Can you work these out from the model? Positions are in its coordinate system, mm. A direction names the side the tool comes from. Round coordinates to 2 decimals unless told otherwise and drop trailing zeros. Order: outer loops, then holes, each group sorted by start corner. A loop starts at its lowest first (then second) coordinate and runs counter-clockwise, first axis right, second up.
from build123d import *

# Parameters (mm, degrees)
EXTRUDE_1_DEPTH      = 12
EXTRUDE_1_DEPTH_BACK = 12
SKETCH_1_W           = 130
SKETCH_1_H           = 112
SKETCH_2_W           = 10.341275007
SKETCH_2_H           = 108.506204724
CUT_EXTRUDE_1_DEPTH  = 90.089842294
SKETCH_3_W           = 108.506204724
SKETCH_3_H           = 4.039795579
SKETCH_3_H_2         = 16.032937215
CUT_EXTRUDE_2_DEPTH  = 5
CHAMFER_1_SIZE       = 5
FILLET_1_R           = 5
CHAMFER_2_SIZE       = 2.747477419
CHAMFER_2_SIZE_2     = 1
FILLET_2_R           = 2
SKETCH_4_W           = 9.4
SKETCH_4_H           = 11
SKETCH_4_W_2         = 7.4
SKETCH_4_H_2         = 9
EXTRUDE_2_DEPTH      = 8
SKETCH_5_W           = 122.805441914
SKETCH_5_H           = 111.758877205
CUT_EXTRUDE_3_DEPTH  = 2


with BuildPart() as part:
    # 草图1 → 凸台-拉伸1 (new, two sides: drawn at the far end of the back side and taken through both)
    with BuildSketch(Plane(origin=(0, 0, 0), x_dir=(1, 0, 0), z_dir=(0, 1, 0)).offset(-EXTRUDE_1_DEPTH_BACK)):
        Rectangle(SKETCH_1_W, SKETCH_1_H)
    extrude(amount=EXTRUDE_1_DEPTH + EXTRUDE_1_DEPTH_BACK)

    # 草图2 → 切除-拉伸1 (cut, through all)
    with BuildSketch(Plane(origin=(0, 12, 0), x_dir=(1, 0, 0), z_dir=(0, 1, 0))):
        with Locations((59.829362496, 1.746897638)):
            Rectangle(SKETCH_2_W, SKETCH_2_H)
        with Locations((-59.829362496, 1.746897638)):
            Rectangle(SKETCH_2_W, SKETCH_2_H)
    extrude(amount=-CUT_EXTRUDE_1_DEPTH, mode=Mode.SUBTRACT)

    # 草图3 → 切除-拉伸2 (cut)
    with BuildSketch(Plane.ZY.offset(54.658724993)):
        with Locations((-1.746897638, 9.980102211)):
            Rectangle(SKETCH_3_W, SKETCH_3_H)
        with Locations((-1.746897638, -3.983531392)):
            Rectangle(SKETCH_3_W, SKETCH_3_H_2)
    cut_extrude_2 = extrude(amount=-CUT_EXTRUDE_2_DEPTH, mode=Mode.SUBTRACT)

    # 镜向1: 切除-拉伸2 across plane
    add(cut_extrude_2.mirror(Plane(origin=(0, 0, 0), x_dir=(0, 0, 1), z_dir=(1, 0, 0))), mode=Mode.SUBTRACT)

    # 倒角1
    chamfer_1_edges = [part.edges().sort_by_distance(p)[0] for p in [
        (-54.658724993, 5.996570818, -56),
        (54.658724993, 5.996570818, -56),
    ]]
    chamfer(chamfer_1_edges, length=CHAMFER_1_SIZE)

    # 圆角1
    # the kernel refuses this fillet: 5 mm, written as the material it takes off along each edge
    with BuildSketch(Plane(origin=(-49.658724993, 12, -68.267336577), x_dir=(0, -1, 0), z_dir=(0, 0, 1))) as fillet_1_piece_1:
        with BuildLine():
            CenterArc((5, 4.906934631), FILLET_1_R, 180, 78.928088112)
            Line((0, 4.906934631), (0, 0))
            Line((0, 0), (4.039795579, 0))
        make_face()
    extrude(amount=120.773541301, mode=Mode.SUBTRACT)
    with BuildSketch(Plane(origin=(-49.658724993, -12, -68.5), x_dir=(0, 1, 0), z_dir=(0, 0, 1)), Plane(origin=(49.658724993, -12, -68.5), x_dir=(-1, 0, 0), z_dir=(0, 0, 1))) as fillet_1_piece_2:
        with BuildLine():
            CenterArc((FILLET_1_R, -FILLET_1_R), FILLET_1_R, 90, 90)
            Line((0, -FILLET_1_R), (0, 0))
            Line((0, 0), (FILLET_1_R, 0))
        make_face()
    extrude(amount=121.006204724, mode=Mode.SUBTRACT)
    with BuildSketch(Plane(origin=(49.658724993, 12, -68.267336577), x_dir=(-1, 0, 0), z_dir=(0, 0, 1))) as fillet_1_piece_3:
        with BuildLine():
            CenterArc((4.906934631, 5), FILLET_1_R, 191.071911888, 78.928088112)
            Line((0, 4.039795579), (0, 0))
            Line((0, 0), (4.906934631, 0))
        make_face()
    extrude(amount=120.773541301, mode=Mode.SUBTRACT)

    # 倒角2
    # the kernel refuses this chamfer: 2.747477419, 1 mm, written as the material it takes off along each edge
    with BuildSketch(Plane(origin=(54.658724993, 7.960204421, 52.506204724), x_dir=(0.013184058198646324, -0.9999130865277316, 0), z_dir=(0, 0, -1))) as chamfer_2_piece_1:
        Polygon((CHAMFER_2_SIZE * 0.999913086693, CHAMFER_2_SIZE * 0.0131840582008), (-CHAMFER_2_SIZE_2 * 0.0131840581986, CHAMFER_2_SIZE_2 * 0.999913086528), (0, 0), align=None)
    extrude(amount=110.633696174, mode=Mode.SUBTRACT)
    with BuildSketch(Plane(origin=(54.658724993, 4.032937215, 52.506204724), x_dir=(-0.9950833631817486, -0.09904090225205064, 0), z_dir=(0, 0, -1))) as chamfer_2_piece_2:
        Polygon((CHAMFER_2_SIZE_2 * 0.995083363182, CHAMFER_2_SIZE_2 * 0.0990409022521), (-CHAMFER_2_SIZE * 0.0990409022684, CHAMFER_2_SIZE * 0.995083363346), (0, 0), align=None)
    extrude(amount=110.633696174, mode=Mode.SUBTRACT)
    with BuildSketch(Plane(origin=(-54.658724993, 4.032937215, 52.506204724), x_dir=(0.9999130865277316, -0.013184058198645857, 0), z_dir=(0, 0, -1))) as chamfer_2_piece_3:
        Polygon((CHAMFER_2_SIZE * 0.999913086693, -CHAMFER_2_SIZE * 0.0131840582008), (-CHAMFER_2_SIZE_2 * 0.0131840581986, -CHAMFER_2_SIZE_2 * 0.999913086528), (0, 0), align=None)
    extrude(amount=110.633696174, mode=Mode.SUBTRACT)
    with BuildSketch(Plane(origin=(-54.658724993, 7.960204421, 52.506204724), x_dir=(-0.09904090225204956, -0.9950833631817488, 0), z_dir=(0, 0, -1))) as chamfer_2_piece_4:
        Polygon((CHAMFER_2_SIZE_2 * 0.995083363182, -CHAMFER_2_SIZE_2 * 0.099040902252), (-CHAMFER_2_SIZE * 0.0990409022684, -CHAMFER_2_SIZE * 0.995083363346), (0, 0), align=None)
    extrude(amount=110.633696174, mode=Mode.SUBTRACT)

    # 圆角2
    fillet_2_edges = [part.edges().sort_by_distance(p)[0] for p in [
        (65, -12, 54.253102362),
        (65, 12, 54.253102362),
        (-65, 12, 54.253102362),
        (-65, -12, 54.253102362),
    ]]
    fillet(fillet_2_edges, radius=FILLET_2_R)

    # 草图4 → 凸台-拉伸2 (add)
    # profile 1 of 9: a face of its own
    with BuildSketch(Plane.XY.offset(56)):
        with Locations((-29.973556768, 0)):
            Rectangle(SKETCH_4_W, SKETCH_4_H)
        with Locations((-29.973556768, 0)):
            Rectangle(SKETCH_4_W_2, SKETCH_4_H_2, mode=Mode.SUBTRACT)
    # profile 2 of 9: a face of its own
    with BuildSketch(Plane.XY.offset(56)):
        with Locations((-41.973556768, 0)):
            Rectangle(SKETCH_4_W, SKETCH_4_H)
        with Locations((-41.973556768, 0)):
            Rectangle(SKETCH_4_W_2, SKETCH_4_H_2, mode=Mode.SUBTRACT)
    # profile 3 of 9: a face of its own
    with BuildSketch(Plane.XY.offset(56)):
        with Locations((-20.073556768, 0)):
            Rectangle(SKETCH_4_W, SKETCH_4_H)
        with Locations((-20.073556768, 0)):
            Rectangle(SKETCH_4_W_2, SKETCH_4_H_2, mode=Mode.SUBTRACT)
    # profile 4 of 9: a face of its own
    with BuildSketch(Plane.XY.offset(56)):
        with Locations((-7.973556768, 0)):
            Rectangle(SKETCH_4_W, SKETCH_4_H)
        with Locations((-7.973556768, 0)):
            Rectangle(SKETCH_4_W_2, SKETCH_4_H_2, mode=Mode.SUBTRACT)
    # profile 5 of 9: a face of its own
    with BuildSketch(Plane.XY.offset(56)):
        with Locations((1.926443232, 0)):
            Rectangle(SKETCH_4_W, SKETCH_4_H)
        with Locations((1.926443232, 0)):
            Rectangle(SKETCH_4_W_2, SKETCH_4_H_2, mode=Mode.SUBTRACT)
    # profile 6 of 9: a face of its own
    with BuildSketch(Plane.XY.offset(56)):
        with Locations((14.026443232, 0)):
            Rectangle(SKETCH_4_W, SKETCH_4_H)
        with Locations((14.026443232, 0)):
            Rectangle(SKETCH_4_W_2, SKETCH_4_H_2, mode=Mode.SUBTRACT)
    # profile 7 of 9: a face of its own
    with BuildSketch(Plane.XY.offset(56)):
        with Locations((23.926443232, 0)):
            Rectangle(SKETCH_4_W, SKETCH_4_H)
        with Locations((23.926443232, 0)):
            Rectangle(SKETCH_4_W_2, SKETCH_4_H_2, mode=Mode.SUBTRACT)
    # profile 8 of 9: a face of its own
    with BuildSketch(Plane.XY.offset(56)):
        with Locations((36.026443232, 0)):
            Rectangle(SKETCH_4_W, SKETCH_4_H)
        with Locations((36.026443232, 0)):
            Rectangle(SKETCH_4_W_2, SKETCH_4_H_2, mode=Mode.SUBTRACT)
    # profile 9 of 9: a face of its own
    with BuildSketch(Plane.XY.offset(56)):
        with Locations((45.926443232, 0)):
            Rectangle(SKETCH_4_W, SKETCH_4_H)
        with Locations((45.926443232, 0)):
            Rectangle(SKETCH_4_W_2, SKETCH_4_H_2, mode=Mode.SUBTRACT)
    extrude(amount=EXTRUDE_2_DEPTH)

    # 草图5 → 切除-拉伸3 (cut)
    with BuildSketch(Plane(origin=(0, 12, 0), x_dir=(1, 0, 0), z_dir=(0, 1, 0))):
        with Locations((1.597279043, 3.373233879)):
            Rectangle(SKETCH_5_W, SKETCH_5_H)
    cut_extrude_3 = extrude(amount=-CUT_EXTRUDE_3_DEPTH, mode=Mode.SUBTRACT)

    # 镜向2: 切除-拉伸3 across plane
    add(cut_extrude_3.mirror(Plane.ZX), mode=Mode.SUBTRACT)


solid = part.part
(1) On a 3-axis mill with a long thin cutter (end or side, diameter ignored), from which of +Z, -Z, +X, -X, +Y, -Y can I reach the whole of each face in a straight line? I mean faces 4 (the face through (2, 5.5, 60)), 5 (the face through (2, 0, 56)), 6 (the face through (-3.274, 0, 60)), 7 (the face through (14, -5.5, 60)), 8 (the face through (20, 0, 64)). Say none if no direction works.
(2) I want a section at A-A, the plane x = 47. List the corners of the cut face in (y, z) for me, plus the area to 3 significant figures.
(3) If we mould it in two halves opening along X, with no side actions, what happens to faces 1 (the face through (65, 0, 54)), 2 (the face through (-1, 12, 54)), 3 (the face through (-37.274, 0, 60))? For each: pulls with the +X half, pulls with the -X half, needs draft (parallel to the pull), parting line crosses it, or undercut.
(4) I'm going to push flat-ended pins straight in: pin 1 Ø4 at (y, z) = (0.5, 58.5) entering from +X; pin 2 Ø4 at (y, z) = (-0.5, 59) entering from -X; pin 3 Ø8 at (y, z) = (-9, 46) entering from +X. Where does each tip first touch, or does it pass through?
(5) Please list where these lines run through material, in increasing order: probe 1 along Z at (x, y) = (56.5, -8.75); probe 2 along Y at (x, z) = (21.5, 58.5); probe 3 along Z at (x, y) = (-46.5, 8.5).
(6) I want a section at B-B, the plane z = 18.5. List the corners of the cut face in (x, y) for me.
Ans:
1. face 4: +Z, +X, -X, +Y
1. face 5: +Z
1. face 6: +Z, +Y, -Y
1. face 7: +Z, +X, -X, -Y
1. face 8: +Z, +X, -X, +Y, -Y
2. outline: (-12, 52.51) - (-10, 52.51) - (-10, -56) - (10, -56) - (10, 52.51) - (12, 52.51) - (12, 56) - (5.5, 56) - (5.5, 64) - (4.5, 64) - (4.5, 56) - (-4.5, 56) - (-4.5, 64) - (-5.5, 64) - (-5.5, 56) - (-12, 56) - close
2. area: 2,270 mm2
3. face 1: pulls with the +X half
3. face 2: needs draft
3. face 3: undercut
4. pin 1: stops at x = 50.63
4. pin 2: stops at x = -46.67
4. pin 3: stops at x = 49.66
5. probe 1: z = 52.51 to 56
5. probe 2: y = -5.5 to -4.5, 4.5 to 5.5
5. probe 3: z = -56 to 56
6. outline: (-54.66, 5.03) - (-51.91, 4.03) - (-49.66, 4.03) - (-49.66, -7) arc R5 ccw to (-48.66, -10) - (48.66, -10) arc R5 ccw to (49.66, -7) - (49.66, 4.03) - (53.66, 4.03) - (54.37, 6) - (53.66, 7.96) - (49.66, 7.96) arc R5 ccw to (48.75, 10) - (-48.75, 10) arc R5 ccw to (-49.66, 7.96) - (-51.91, 7.96) - (-54.66, 6.96) - close
